Could you check a few things on this model? Use its own coordinates, in mm. Face numbers are marked on the shaded views. A direction names the side the tool comes from. Round coordinates to 2 decimals unless told otherwise and drop trailing zeros. Loops run counter-clockwise (first coordinate to the right, second up) from the corner with the lowest first, then second, coordinate; pieces in that order, holes last. Notation, with made-up numbers: (43.5, -29) -> (80.5, -29) arc R20 ccw to (80.5, -19) -> close; hole circle Ø2 at (46.5, 89). An arc over 180 degrees is marked (long way). One line per item, written item: value.
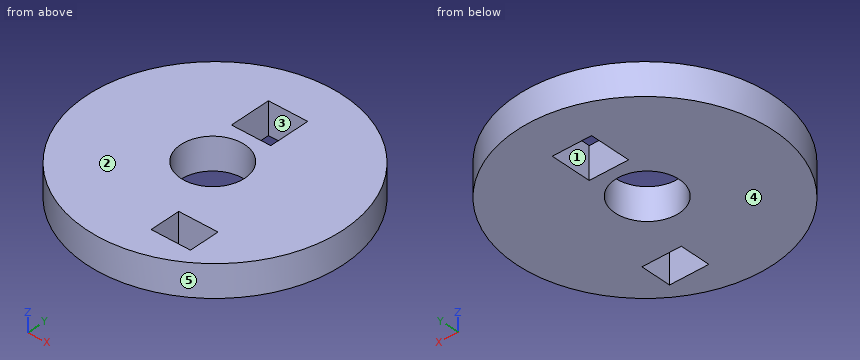
```python
from build123d import *

# Parameters (mm, degrees)
F0_R     = 50.8
F0_R_2   = 12.7
F0_W     = 15.568451
F0_H     = 12.218274
F0_W_2   = 15.568449
F0_H_2   = 16.356724
F1_DEPTH = 12.7


with BuildPart() as f1:
    # F0 (on Top) → F1 (new body)
    with BuildSketch(Plane.XY):
        with Locations((0.908604, 0)):
            Circle(F0_R)
        Circle(F0_R_2, mode=Mode.SUBTRACT)
        with Locations((17.046467, -31.531036)):
            Rectangle(F0_W, F0_H, mode=Mode.SUBTRACT)
        with Locations((-0.295603, 25.520432)):
            Rectangle(F0_W_2, F0_H_2, mode=Mode.SUBTRACT)
    extrude(amount=F1_DEPTH)


solid = f1.part
```
Item 1: If we section it at C-C on x = -10: List the corners of the cut face in (y, z) for me, plus the area to 3 significant figures.
Output:
outline: (-49.61, 0) -> (-7.83, 0) -> (-7.83, 12.7) -> (-49.61, 12.7) -> close; (7.83, 0) -> (49.61, 0) -> (49.61, 12.7) -> (7.83, 12.7) -> close
area: 1,060 mm²
Item 2: Will these pins go through, and if not, where does the flat tip stop? pin 1 Ø6 at (y, z) = (-30.5, 3.5) entering from +X; pin 2 Ø1 at (y, z) = (20.5, 10.5) entering from -X; pin 3 Ø4 at (x, z) = (-14, 1.5) entering from +Y; pin 4 Ø10 at (x, y) = (-14, -4.5) entering from -Z.
Output:
pin 1: stops at x = 43.62
pin 2: stops at x = -45.79
pin 3: stops at y = 49.13
pin 4: stops at z = 0
Item 3: If we section it at D-D on x = -35: List the corners of the cut face in (y, z) for me, plus the area to 3 significant figures.
Output:
outline: (-35.93, 0) -> (35.93, 0) -> (35.93, 12.7) -> (-35.93, 12.7) -> close
area: 913 mm²
Item 4: If we mould it in two halves opening along Y, with no side actions, what happens to the marked faces 3, 4 and 5? For each: released by +Y, released by -Y, zero draft, split by the parting line, or undercut.
Output:
face 3: undercut
face 4: zero draft
face 5: split by the parting line
Item 5: For the marked faces 1 and 2, which set-ups out of +Z, -Z, +X, -X, +Y, -Y let a thin tool reach every point of the face, with its end or its side?
Output:
face 1: +Z, -Z
face 2: +Z, +X, -X, +Y, -Y
Item 6: I need wall thicknesses on line 1 (Y direction, x = 0, z = 7); line 2 (Y direction, x = -6, z = 7.25); line 3 (Y direction, x = 16, z = 5.5). Which ranges of each line are inside material? Lowest first, please. Write a range as from..to.
Output:
line 1: y = -50.79..-12.7, 12.7..17.34, 33.7..50.79
line 2: y = -50.33..-11.19, 11.19..17.34, 33.7..50.33
line 3: y = -48.51..-37.64, -25.42..48.51
Item 7: If we section it at B-B on z = 7: List the corners of the cut face in (x, y) for me, plus the area to 3 significant figures.
Output:
outline: circle Ø101.6 at (0.91, 0); hole circle Ø25.4 at (0, 0); hole (-8.08, 17.34) -> (7.49, 17.34) -> (7.49, 33.7) -> (-8.08, 33.7) -> close; hole (9.26, -37.64) -> (24.83, -37.64) -> (24.83, -25.42) -> (9.26, -25.42) -> close
area: 7,160 mm²
Item 8: If we section it at A-A on y = 0: List the corners of the cut face in (x, z) for me, plus the area to 3 significant figures.
Output:
outline: (-49.89, 0) -> (-12.7, 0) -> (-12.7, 12.7) -> (-49.89, 12.7) -> close; (12.7, 0) -> (51.71, 0) -> (51.71, 12.7) -> (12.7, 12.7) -> close
area: 968 mm²
